Here's how the part is built. I have some questions about the finished solid (model axes, mm). Face numbers are marked on the shaded views. A direction names the side the tool comes from. Give positions to 0.01 mm unless a question says otherwise; leave off trailing zeros. Loops run counter-clockwise (first coordinate to the right, second up) from the corner with the lowest first, then second, coordinate; pieces in that order, holes last. Notation, with made-up numbers: M -34.5,76.5 L 20.5,76.5 A15 ccw 20.5,94.5 Z; hole C 49,-21.5 d10. An arc over 180 degrees is marked long. Write item = value, one per line. Start each with the question number.
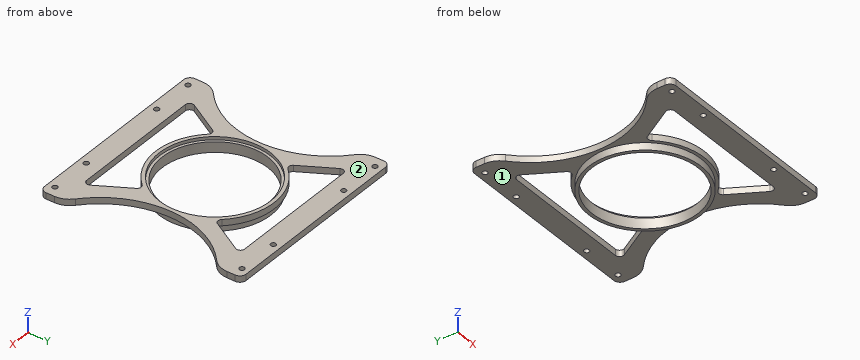
```python
from build123d import *

# Parameters (mm, degrees)
SKETCH006_R     = 27
SKETCH006_R_2   = 25.45
PAD003_DEPTH    = 3.5
SKETCH007_W     = 95
SKETCH007_H     = 97
SKETCH007_R     = 25.45
PAD004_DEPTH    = 3
SKETCH008_R     = 26.765
POCKET_DEPTH    = 1.5
SKETCH009_R     = 1.25
POCKET001_DEPTH = 6.501
SKETCH010_R     = 45
POCKET002_DEPTH = 6.501
FILLET_R        = 10
FILLET001_R     = 3


with BuildPart() as part:
    # Sketch006 → Pad003 (new body)
    with BuildSketch(Plane.XY):
        Circle(SKETCH006_R)
        Circle(SKETCH006_R_2, mode=Mode.SUBTRACT)
    extrude(amount=PAD003_DEPTH)

    # Sketch007 (on Face4 of Pad003) → Pad004 (join)
    with BuildSketch(Plane.XY.offset(3.5)):
        Rectangle(SKETCH007_W, SKETCH007_H)
        Circle(SKETCH007_R, mode=Mode.SUBTRACT)
    extrude(amount=PAD004_DEPTH)

    # Sketch008 (on Face10 of Pad004) → Pocket (cut)
    with BuildSketch(Plane.XY.offset(6.5)):
        Circle(SKETCH008_R)
    extrude(amount=-POCKET_DEPTH, mode=Mode.SUBTRACT)

    # Sketch009 (on Face10 of Pocket) → Pocket001 (cut, through all)
    with BuildSketch(Plane.XY.offset(6.5)):
        with Locations((-42.5, 45)):
            Circle(SKETCH009_R)
        with Locations((42.5, 45)):
            Circle(SKETCH009_R)
        with Locations((42.5, -45)):
            Circle(SKETCH009_R)
        with Locations((-42.5, -45)):
            Circle(SKETCH009_R)
        with Locations((-22.5, 45)):
            Circle(SKETCH009_R)
        with Locations((22.5, 45)):
            Circle(SKETCH009_R)
        with Locations((-22.5, -45)):
            Circle(SKETCH009_R)
        with Locations((22.5, -45)):
            Circle(SKETCH009_R)
    extrude(amount=-POCKET001_DEPTH, mode=Mode.SUBTRACT)

    # Sketch010 (on Face18 of Pocket001) → Pocket002 (cut, through all)
    with BuildSketch(Plane.XY.offset(6.5)):
        with Locations((-73.5, 0)):
            Circle(SKETCH010_R)
        with Locations((73.5, 0)):
            Circle(SKETCH010_R)
        with BuildLine():
            Line((-31.535898, 38), (31.535898, 38))
            ThreePointArc((33.267949, 35), (33.267949, 37), (31.535898, 38))
            Line((33.267949, 35), (24.317547, 19.497448))
            ThreePointArc((21.10448, 19.153353), (22.798463, 18.508819), (24.317547, 19.497448))
            ThreePointArc((21.10448, 19.153353), (0, 28.5), (-21.10448, 19.153353))
            ThreePointArc((-24.317547, 19.497448), (-22.798463, 18.508819), (-21.10448, 19.153353))
            Line((-33.267949, 35), (-24.317547, 19.497448))
            ThreePointArc((-31.535898, 38), (-33.267949, 37), (-33.267949, 35))
        make_face()
        with BuildLine():
            Line((-31.535898, -38), (31.535898, -38))
            ThreePointArc((31.535898, -38), (33.267949, -37), (33.267949, -35))
            Line((33.267949, -35), (24.317547, -19.497448))
            ThreePointArc((24.317547, -19.497448), (22.798463, -18.508819), (21.10448, -19.153353))
            ThreePointArc((-21.10448, -19.153353), (0, -28.5), (21.10448, -19.153353))
            ThreePointArc((-21.10448, -19.153353), (-22.798463, -18.508819), (-24.317547, -19.497448))
            Line((-33.267949, -35), (-24.317547, -19.497448))
            ThreePointArc((-33.267949, -35), (-33.267949, -37), (-31.535898, -38))
        make_face()
    extrude(amount=-POCKET002_DEPTH, mode=Mode.SUBTRACT)

    # Fillet
    fillet_edges = [part.edges().sort_by_distance(p)[0] for p in [
        (47.5, -36.728735, 5),
        (47.5, 36.728735, 5),
        (-47.5, -36.728735, 5),
        (-47.5, 36.728735, 5),
    ]]
    fillet(fillet_edges, radius=FILLET_R)

    # Fillet001
    fillet001_edges = [part.edges().sort_by_distance(p)[0] for p in [
        (-47.5, 48.5, 5),
        (-47.5, -48.5, 5),
        (47.5, 48.5, 5),
        (47.5, -48.5, 5),
    ]]
    fillet(fillet001_edges, radius=FILLET001_R)


solid = part.part
```
Q1. If we section it at B-B, the plane x = 0: List the corners of the cut face in (y, z) for me (3 decimals).
Q2. If we section it at D-D, the plane z = 1: List the corners of the cut face in (x, y) for me.
Q3. If I drill on line 1 along Y through (x, z) = (-1, 5.75); line 2 along Y through (x, z) = (42.5, 4.7); line 3 along Y through (x, z) = (22.5, 4.9), over which ranges is the centre line in solid material (lowest first)?
Q4. If we section it at A-A, the plane y = 0: List the corners of the cut face in (x, z) for me (3 decimals), then the cut area to 3 significant figures.
Q5. Will these pins go through, and if not, where does the flat tip stop? pin 1 (3 mm diameter, centred on x = -5, z = 1, fed in from +Y); pin 2 (16 mm diameter, centred on x = 11.5, y = 7.5, fed in from +Z); pin 3 (1.5 mm diameter, centred on y = -5, z = 4.5, fed in from +X); pin 4 (4 mm diameter, centred on x = -22.5, y = -45, fed in from -Z).
Q6. If we section it at C-C, the plane x = -22.5: State how many separate pieces and enclosed holes the cut face has, then the cut area to 3 significant figures.
Q7. On a 3-axis mill with a long thin cutter (end or side, diameter ignored), from which of +Z, -Z, +X, -X, +Y, -Y can I reach the whole of each face in a straight line? I mean the marked faces 1 and 2. Say none if no direction works.
Resolved:
q1.outline = M -48.5,3.5 L -38,3.5 L -38,6.5 L -48.5,6.5 Z; M -28.5,3.5 L -27,3.5 L -27,0 L -25.45,0 L -25.45,5 L -26.765,5 L -26.765,6.5 L -28.5,6.5 Z; M 25.45,0 L 27,0 L 27,3.5 L 28.5,3.5 L 28.5,6.5 L 26.765,6.5 L 26.765,5 L 25.45,5 Z; M 38,3.5 L 48.5,3.5 L 48.5,6.5 L 38,6.5 Z
q2.outline = C 0,0 d54; hole C 0,0 d50.9
q3.line_1 = -48.5 to -38, -28.48 to -26.75, 26.75 to 28.48, 38 to 48.5
q3.line_2 = -48.5 to -46.25, -43.75 to -32.62, 32.62 to 43.75, 46.25 to 48.5
q3.line_3 = -48.5 to -46.25, -43.75 to -38, -18.5 to -11.89, 11.89 to 18.5, 38 to 43.75, 46.25 to 48.5
q4.outline = M -28.5,3.5 L -27,3.5 L -27,0 L -25.45,0 L -25.45,5 L -26.765,5 L -26.765,6.5 L -28.5,6.5 Z; M 25.45,0 L 27,0 L 27,3.5 L 28.5,3.5 L 28.5,6.5 L 26.765,6.5 L 26.765,5 L 25.45,5 Z
q4.area = 25.2 mm²
q5.pin_1 = 26.77
q5.pin_2 = through
q5.pin_3 = 28.87
q5.pin_4 = 3.5
q6.separate_pieces = 6
q6.enclosed_holes = 0
q6.area = 101 mm²
q7.face_1 = -Z
q7.face_2 = +Z, +X, -X, +Y, -Y
